Here's how the part is built. I have some questions about the finished solid (model axes, mm). A direction names the side the tool comes from. Coordinates: 2 decimals unless noted, no trailing zeros. Write each loop counter-clockwise with the first axis right and the second up, starting at its lowest first coordinate (ties: lowest second). Pieces come first, ordered by that corner, then holes.
(1) Thinking about a two-plate mould opening in Y: for faces 5 (the flat face through (-0.3, 0, -11.3)), 6 (the flat face through (16, 40, -14)), 7 (the flat face through (-12, 40, 3)), which applies, released by +Y, released by -Y, zero draft, split by the parting line, or undercut?
(2) Imagine slicing it at D-D, the plane y = 62. State how many separate pieces and enclosed holes the cut face has, plus the area to 3 significant figures.
(3) Imagine slicing it at A-A, the plane y = 45. List the corners of the cut face in (x, z) for me, plus the area to 3 significant figures.
(4) Imagine slicing it at C-C, the plane x = 0. List the corners of the cut face in (y, z) for me.
(5) Imagine slicing it at B-B, the plane z = -16.5. List the corners of the cut face in (x, y) for me.
(6) Please list where these lines run through material, in increasing order: probe 1 along X at (y, z) = (37, -9.75); probe 2 along Y at (x, z) = (-17, -6.5); probe 3 along X at (y, z) = (45, -5.25).
(7) Which directions (+Z, -Z, +X, -X, +Y, -Y) give clear straight access to the entire face, cutting with the end or side of a thin tool? Please do faces 1 (the flat face through (-15, 21, 2)), 2 (the flat face through (-13, 66, 2)), 3 (the flat face through (14, 80, -6)), 4 (the flat face through (0, 78, -15)).
(8) For pin 1 Ø1.8 at (y, z) = (56, -15.5) entering from -X; pin 2 Ø1.3 at (y, z) = (18.5, 1) entering from +X; pin 3 Ø2 at (y, z) = (65, 0.5) entering from -X, each with a flat end and sliding along its axis, tell me the tip position at first contact or that it passes through.
```python
from build123d import *

# Parameters (mm, degrees)
BOSS_EXTRUDE1_DEPTH     = 82
CUT_EXTRUDE1_DEPTH      = 30
CUT_EXTRUDE1_DEPTH_BACK = 30
SKETCH2_W               = 6
SKETCH2_H               = 2
SHELL1_START            = 4
SHELL1_DEPTH            = 74
SHELL1_START_2          = 2
SHELL1_2_DEPTH          = 78
CUT_EXTRUDE2_DEPTH      = 6
CUT_EXTRUDE2_DEPTH_BACK = 6
SKETCH3_W               = 4
SKETCH3_H               = 10
SKETCH4_W               = 13.166010488
SKETCH4_H               = 28
CUT_EXTRUDE3_DEPTH      = 20


# Read off the part's stored shape, not the designer's step: Shell1
with BuildPart() as part:
    # Sketch1 → Boss-Extrude1 (new body)
    with BuildSketch(Plane(origin=(0, 0, 0), x_dir=(1, 0, 0), z_dir=(0, 1, 0))):
        with BuildLine():
            Line((-20, 12), (-20, 3))
            ThreePointArc((-20, 3), (-18.242640687, -1.242640687), (-14, -3))
            Line((-14, -3), (-10.583005244, -3))
            ThreePointArc((-10.583005244, -3), (0, 11), (10.583005244, -3))
            Line((10.583005244, -3), (14, -3))
            ThreePointArc((14, -3), (18.242640687, -1.242640687), (20, 3))
            Line((20, 3), (20, 12))
            Line((20, 12), (18, 12))
            Line((18, 12), (18, 18))
            Line((18, 18), (-18, 18))
            Line((-18, 18), (-18, 12))
            Line((-18, 12), (-20, 12))
        make_face()
    extrude(amount=BOSS_EXTRUDE1_DEPTH)

    # Sketch2 → Cut-Extrude1 (cut, two sides: drawn at the far end of the back side and taken through both)
    with BuildSketch(Plane(origin=(0, 0, 0), x_dir=(0, 0, -1), z_dir=(1, 0, 0)).offset(-CUT_EXTRUDE1_DEPTH_BACK)):
        with Locations((15, 81)):
            Rectangle(SKETCH2_W, SKETCH2_H)
        with Locations((15, 1)):
            Rectangle(SKETCH2_W, SKETCH2_H)
    extrude(amount=CUT_EXTRUDE1_DEPTH + CUT_EXTRUDE1_DEPTH_BACK, mode=Mode.SUBTRACT)

    # Shell1 outline → Shell1 (cut)
    with BuildSketch(Plane(origin=(0, 0, 0), x_dir=(1, 0, 0), z_dir=(0, 1, 0)).offset(SHELL1_START)):
        with BuildLine():
            Line((-14, -1), (-12.961481397, -1))
            ThreePointArc((-12.961481397, -1), (0, 13), (12.961481397, -1))
            Line((12.961481397, -1), (14, -1))
            ThreePointArc((14, -1), (16.828427125, 0.171572875), (18, 3))
            Line((18, 3), (18, 10))
            Line((18, 10), (16, 10))
            Line((16, 10), (16, 18))
            Line((16, 18), (-16, 18))
            Line((-16, 18), (-16, 10))
            Line((-16, 10), (-18, 10))
            Line((-18, 10), (-18, 3))
            ThreePointArc((-18, 3), (-16.828427125, 0.171572875), (-14, -1))
        make_face()
    extrude(amount=SHELL1_DEPTH, mode=Mode.SUBTRACT)

    # Shell1 2 outline → Shell1 2 (cut)
    with BuildSketch(Plane(origin=(0, 0, 0), x_dir=(1, 0, 0), z_dir=(0, 1, 0)).offset(SHELL1_START_2)):
        with BuildLine():
            Line((-14, -1), (-12.961481397, -1))
            ThreePointArc((-12.961481397, -1), (-11.972179223, 5.066253514), (-8.306623863, 10))
            Line((-8.306623863, 10), (-18, 10))
            Line((-18, 10), (-18, 3))
            ThreePointArc((-18, 3), (-16.828427125, 0.171572875), (-14, -1))
        make_face()
        with BuildLine():
            Line((18, 10), (8.306623863, 10))
            ThreePointArc((8.306623863, 10), (11.972179223, 5.066253514), (12.961481397, -1))
            Line((12.961481397, -1), (14, -1))
            ThreePointArc((14, -1), (16.828427125, 0.171572875), (18, 3))
            Line((18, 3), (18, 10))
        make_face()
    extrude(amount=SHELL1_2_DEPTH, mode=Mode.SUBTRACT)

    # Sketch3 → Cut-Extrude2 (cut, two sides: drawn at the far end of the back side and taken through both)
    with BuildSketch(Plane.XY.offset(-CUT_EXTRUDE2_DEPTH_BACK)):
        with Locations((-15, 16)):
            Rectangle(SKETCH3_W, SKETCH3_H)
        with Locations((15, 16)):
            Rectangle(SKETCH3_W, SKETCH3_H)
        with Locations((15, 66)):
            Rectangle(SKETCH3_W, SKETCH3_H)
        with Locations((-15, 66)):
            Rectangle(SKETCH3_W, SKETCH3_H)
    extrude(amount=CUT_EXTRUDE2_DEPTH + CUT_EXTRUDE2_DEPTH_BACK, mode=Mode.SUBTRACT)

    # Sketch4 → Cut-Extrude3 (cut)
    with BuildSketch(Plane.XY):
        with Locations((0, 41)):
            Rectangle(SKETCH4_W, SKETCH4_H)
    extrude(amount=-CUT_EXTRUDE3_DEPTH, mode=Mode.SUBTRACT)


solid = part.part
```
Recorded:
1. face 5: released by -Y
1. face 6: undercut
1. face 7: zero draft
2. separate pieces: 3
2. enclosed holes: 0
2. area: 175 mm2
3. outline: (-20, -12) - (-18, -12) - (-18, -18) - (-16, -18) - (-16, -10) - (-18, -10) - (-18, -3) arc R4 cw to (-14, 1) - (-12.96, 1) arc R13 ccw to (-6.58, -11.21) - (-6.58, -8.81) arc R11 cw to (-10.58, 3) - (-14, 3) arc R6 ccw to (-20, -3) - close; (6.58, -11.21) arc R13 ccw to (12.96, 1) - (14, 1) arc R4 cw to (18, -3) - (18, -10) - (16, -10) - (16, -18) - (18, -18) - (18, -12) - (20, -12) - (20, -3) arc R6 ccw to (14, 3) - (10.58, 3) arc R11 cw to (6.58, -8.81) - close
3. area: 164 mm2
4. outline: (0, -12) - (2, -12) - (2, -18) - (4, -18) - (4, -13) - (27, -13) - (27, -11) - (0, -11) - close; (55, -13) - (78, -13) - (78, -18) - (80, -18) - (80, -12) - (82, -12) - (82, -11) - (55, -11) - close
5. outline: (-18, 2) - (18, 2) - (18, 80) - (-18, 80) - close; hole (-16, 4) - (16, 4) - (16, 78) - (-16, 78) - close
6. probe 1: x = -20 to -18, -8.6 to -6.58, 6.58 to 8.6, 18 to 20
6. probe 2: y = 0 to 2, 80 to 82
6. probe 3: x = -20 to -18, -11.89 to -9.67, 9.67 to 11.89, 18 to 20
7. face 1: +Z
7. face 2: +Z, -Z
7. face 3: none
7. face 4: -Z
8. pin 1: stops at x = -18
8. pin 2: stops at x = 18.98
8. pin 3: stops at x = -19.45
